Here's how the part is built. I have some questions about the finished solid (model axes, mm). A direction names the side the tool comes from. Round coordinates to 2 decimals unless told otherwise and drop trailing zeros. Loops run counter-clockwise (first coordinate to the right, second up) from the corner with the lowest first, then second, coordinate; pieces in that order, holes last. Notation, with made-up numbers: (62, 59.5) - (111, 59.5) arc R18 ccw to (111, 91.5) - close; hole circle Ø2 at (82, 30.5). An arc over 180 degrees is marked (long way). Answer as a JSON object with one key per item and string values. Group by question number.
1) If we mould it in two halves opening along Z, with no side actions, what happens to faces 3 (the face through (8, -10, 12.25)), 4 (the face through (1, -10, 0)), 5 (the face through (7.61, -9.86, 11.25))? For each: pulls with the +Z half, pulls with the -Z half, needs draft (parallel to the pull), parting line crosses it, or undercut.
2) I want a section at C-C, the plane z = 6. Please give me the cut outline in (x, y), then the cut area to 3 significant figures.
3) I want a section at B-B, the plane y = -8.25. Please give me the cut outline in (x, z).
4) Which directions (+Z, -Z, +X, -X, +Y, -Y) give clear straight access to the entire face, cutting with the end or side of a thin tool? Please do faces 1 (the face through (15.5, -10, 3)), 2 (the face through (1.5, -10, 3)).
5) I want a section at A-A, the plane z = 2.5. Please give me the cut outline in (x, y).
6) I want a section at D-D, the plane x = 7.75. Please give me the cut outline in (y, z).
7) If I drill on line 1 along X through (y, z) = (-2.5, 3.25); line 2 along X through (y, z) = (-9.25, 0.5); line 3 along Z through (x, y) = (14.75, -17), over which ranges is the centre line in solid material (lowest first)? Write a range as [from, to].
8) Will these pins go through, and if not, where does the flat tip stop? P1, Ø1.5, axis at y = -14.5, z = 8, coming from the -X side; P2, Ø3, axis at x = 4.5, y = -5, coming from the -Z side; P3, Ø1.5, axis at x = 3, z = 5, coming from the +Y side.
from build123d import *

# Parameters (mm, degrees)
F1_DEPTH = 20


with BuildPart() as f1:
    # F0 (on Front) → F1 (new body)
    with BuildSketch(Plane.XZ):
        with BuildLine():
            Line((0, 7), (0, 0))
            Line((0, 0), (1.5, 0))
            Line((1.5, 0), (2, 0.2))
            Line((2, 0.2), (2, 0.75))
            Line((2, 0.75), (1.5, 0.75))
            Line((1.5, 0.75), (1.5, 5))
            ThreePointArc((1.5, 5), (7.75, 11.25), (14, 5))
            Line((14, 5), (14, 0.75))
            Line((14, 0.75), (13.5, 0.75))
            Line((13.5, 0.75), (13.5, 0.2))
            Line((13.5, 0.2), (14, 0))
            Line((14, 0), (15.5, 0))
            Line((15.5, 0), (15.5, 7))
            Line((15.5, 7), (11.166384, 12.25))
            Line((11.166384, 12.25), (7.75, 12.25))
            Line((7.75, 12.25), (4.333616, 12.25))
            Line((4.333616, 12.25), (0, 7))
        make_face()
    extrude(amount=F1_DEPTH)


solid = f1.part
Outcome:
{
 "1": {"face 3": "pulls with the +Z half", "face 4": "pulls with the -Z half", "face 5": "undercut"},
 "2": {"outline": "(0, -20) - (1.58, -20) - (1.58, 0) - (0, 0) - close; (13.92, -20) - (15.5, -20) - (15.5, 0) - (13.92, 0) - close", "area": "63.2 mm^2"},
 "3": {"outline": "(0, 0) - (1.5, 0) - (2, 0.2) - (2, 0.75) - (1.5, 0.75) - (1.5, 5) arc R6.25 cw to (14, 5) - (14, 0.75) - (13.5, 0.75) - (13.5, 0.2) - (14, 0) - (15.5, 0) - (15.5, 7) - (11.17, 12.25) - (4.33, 12.25) - (0, 7) - close"},
 "4": {"face 1": "+Z, -Z, +X, +Y, -Y", "face 2": "+Y, -Y"},
 "5": {"outline": "(0, -20) - (1.5, -20) - (1.5, 0) - (0, 0) - close; (14, -20) - (15.5, -20) - (15.5, 0) - (14, 0) - close"},
 "6": {"outline": "(-20, 11.25) - (0, 11.25) - (0, 12.25) - (-20, 12.25) - close"},
 "7": {"line 1": "[0, 1.5], [14, 15.5]", "line 2": "[0, 2], [13.5, 15.5]", "line 3": "[0, 7.91]"},
 "8": {"P1": "x = 0.21", "P2": "z = 9.06", "P3": "through"}
}
